```python
from build123d import *

# Parameters (mm, degrees)
F0_W     = 83.566
F0_H     = 55.9689
F1_DEPTH = 10.9093
F2_W     = 83.566
F2_H     = 31.1531
F3_DEPTH = 14.1097
F4_W     = 50.8889
F4_H     = 46.1518
F5_DEPTH = 4.699
F6_W     = 43.3959
F6_H     = 24.9174
F7_DEPTH = 20.0152
F8_R     = 5.55625
F9_DEPTH = 25.4


with BuildPart() as f1:
    # F0 (on Front) → F1 (new body)
    with BuildSketch(Plane.XZ):
        Rectangle(F0_W, F0_H)
    extrude(amount=F1_DEPTH)

    # F2 (on face) → F3 (join)
    with BuildSketch(Plane(origin=(0, 0, 0), x_dir=(-1, 0, 0), z_dir=(0, 1, 0))):
        with Locations((0, -12.4079)):
            Rectangle(F2_W, F2_H)
    extrude(amount=F3_DEPTH)

    # F4 (on face) → F5 (join)
    with BuildSketch(Plane(origin=(0, 14.1097, 0), x_dir=(-1, 0, 0), z_dir=(0, 1, 0))):
        with Locations((-0.00635, -51.06035)):
            Rectangle(F4_W, F4_H)
    extrude(amount=-F5_DEPTH)

    # F6 (on face) → F7 (cut)
    with BuildSketch(Plane.XZ.offset(10.9093)):
        with Locations((-6.99135, -12.82065)):
            Rectangle(F6_W, F6_H)
    extrude(amount=-F7_DEPTH, mode=Mode.SUBTRACT)

    # F8 (on face) → F9 (cut)
    with BuildSketch(Plane(origin=(0, 14.1097, 0), x_dir=(-1, 0, 0), z_dir=(0, 1, 0))):
        with Locations((18.68805, -13.991897)):
            Circle(F8_R)
    extrude(amount=-F9_DEPTH, mode=Mode.SUBTRACT)


solid = f1.part
```
Work out the finished part from the listing and answer in its coordinate system (mm). A direction names the side the tool comes from. Coordinates: 2 decimals unless noted, no trailing zeros. Write each loop counter-clockwise with the first axis right and the second up, starting at its lowest first coordinate (ties: lowest second). Pieces come first, ordered by that corner, then holes.
Q1. Which of the six approach directions +Z, -Z, +X, -X, +Y, -Y give full straight-line access (tool end or side, diameter ignored) to faces 4 (the face through (25.451, 12, -51)), 5 (the face through (0, 9.411, -51)), 6 (the face through (-7, 9.106, -13)), 7 (the face through (1, 7, 3.169))?
Q2. A cutting plane is placed at A-A, the plane y = -7.25. Give the vertices of the cut face in (x, z).
Q3. A cutting plane is placed at D-D, the plane z = -30. Give the vertices of the cut face in (x, y), then the cut area to 3 significant figures.
Q4. Determine the mould class of faces 1 (the face through (-1, -5, 27.984)), 2 (the face through (-7, -1, -0.362)), 3 (the face through (-25.438, 12, -51)) for opening direction Z: released by +Z, released by -Z, zero draft, split by the parting line, or undercut.
Q5. Each of these flat-tipped pins is pushed along its axis until it touches: pin 1 Ø10 at (x, y) = (3.5, -5.5) entering from -Z; pin 2 Ø4 at (y, z) = (11.5, -44.5) entering from -X; pin 3 Ø4 at (x, y) = (-0.5, 9) entering from +Z. Where does it stop, or does it pass through?
Q6. Find the intervals of material crossed by line 1 (X direction, y = 5, z = -1.5); line 2 (Z direction, x = -9, y = 6.75); line 3 (Z direction, x = -27, y = -3.25), in increasing order.
Q7. A cutting plane is placed at C-C, the plane x = -19. Give the vertices of the cut face in (y, z), then the cut area to 3 significant figures.
Q8. A cutting plane is placed at B-B, the plane x = 1.5. Give the vertices of the cut face in (y, z).
Findings below:
1. face 4: -Z, +X, +Y, -Y
1. face 5: -Z, +X, -X, -Y
1. face 6: -Y
1. face 7: +Z, +X, -X, +Y
2. outline: (-41.78, -27.98) - (41.78, -27.98) - (41.78, 27.98) - (-41.78, 27.98) - close; hole (-28.69, -25.28) - (14.71, -25.28) - (14.71, -0.36) - (-28.69, -0.36) - close
3. outline: (-25.44, 9.41) - (25.45, 9.41) - (25.45, 14.11) - (-25.44, 14.11) - close
3. area: 239 mm2
4. face 1: released by +Z
4. face 2: undercut
4. face 3: zero draft
5. pin 1: stops at z = -27.98
5. pin 2: stops at x = -25.44
5. pin 3: stops at z = 3.17
6. line 1: x = -41.78 to -28.69, 14.71 to 41.78
6. line 2: z = -27.98 to -25.28, -0.36 to 3.17
6. line 3: z = -27.98 to -25.28, -0.36 to 27.98
7. outline: (-10.91, -27.98) - (9.41, -27.98) - (9.41, -74.14) - (14.11, -74.14) - (14.11, -19.54) - (9.11, -19.54) - (9.11, -25.28) - (-10.91, -25.28) - close; (-10.91, -0.36) - (9.11, -0.36) - (9.11, -8.44) - (14.11, -8.44) - (14.11, 3.17) - (0, 3.17) - (0, 27.98) - (-10.91, 27.98) - close
7. area: 713 mm2
8. outline: (-10.91, -27.98) - (9.41, -27.98) - (9.41, -74.14) - (14.11, -74.14) - (14.11, 3.17) - (0, 3.17) - (0, 27.98) - (-10.91, 27.98) - (-10.91, -0.36) - (9.11, -0.36) - (9.11, -25.28) - (-10.91, -25.28) - close
